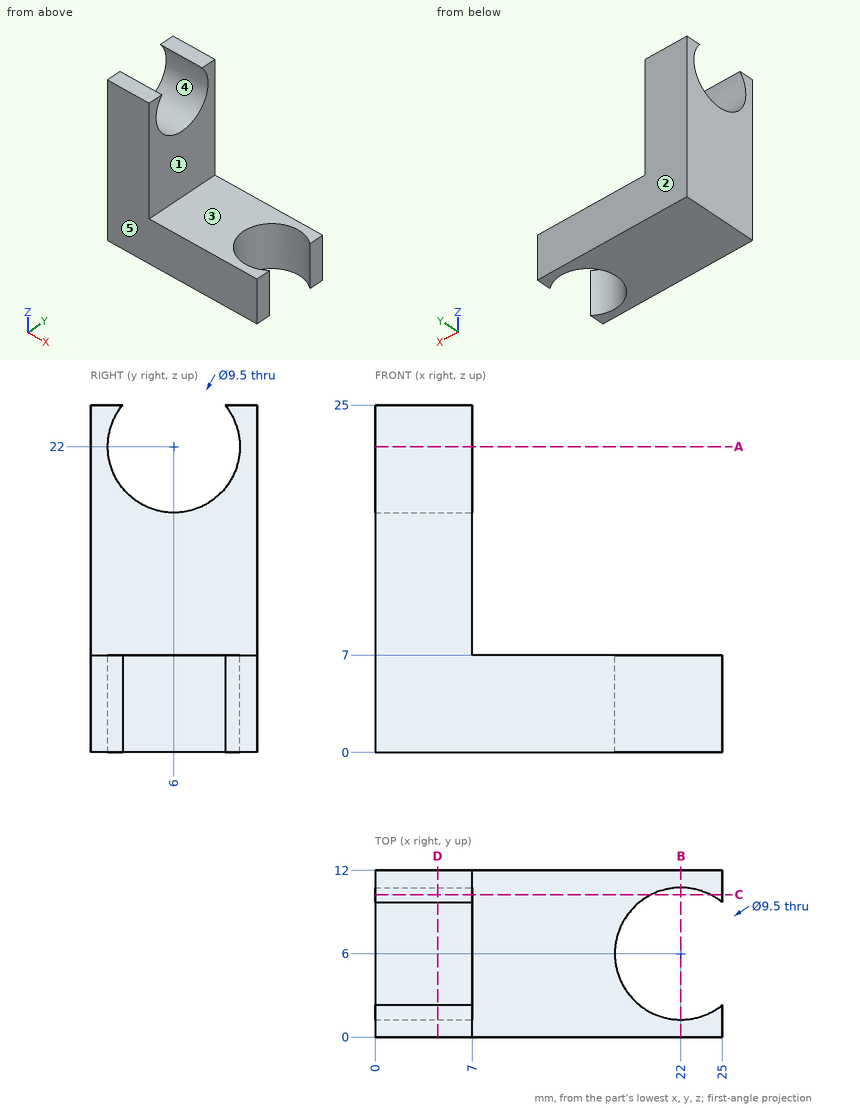
Answer from the drawing. Dimensions are ordinates in mm from the lowest x, y and z of the part. A direction names the side the tool comes from. Give positions to 0.01 mm unless a question says otherwise; leave off trailing zeros. Loops run counter-clockwise (first coordinate to the right, second up) from the corner with the lowest first, then second, coordinate; pieces in that order, holes last. Notation, with made-up numbers: (-22.75, 62) -> (15.25, 62) arc R17 ccw to (15.25, 84) -> close; hole circle Ø10 at (36, 55). An arc over 180 degrees is marked (long way). Use a Markdown table: item, result.
Q1. Section C-C, the plane y = 10.25 is taken. Determine the outline of the cut face in (x, z).
Solved:
| item | result |
|---|---|
| outline | (0, 0) -> (19.88, 0) -> (19.88, 7) -> (7, 7) -> (7, 19.88) -> (0, 19.88) -> close; (0, 24.12) -> (7, 24.12) -> (7, 25) -> (0, 25) -> close; (24.12, 0) -> (25, 0) -> (25, 7) -> (24.12, 7) -> close |
Q2. Section A-A, the plane z = 22 is taken. Determine the outline of the cut face in (x, y).
Solved:
| item | result |
|---|---|
| outline | (0, 0) -> (7, 0) -> (7, 1.25) -> (0, 1.25) -> close; (0, 10.75) -> (7, 10.75) -> (7, 12) -> (0, 12) -> close |
Q3. Find the intervals of material crossed by line 1 along Y through (x, z) = (3.25, 22); line 2 along X through (y, z) = (6, 17), in increasing order.
Solved:
| item | result |
|---|---|
| line 1 | y = 0 to 1.25, 10.75 to 12 |
| line 2 | x = 0 to 7 |
Q4. Section D-D, the plane x = 4.5 is taken. Determine the outline of the cut face in (y, z), then the cut area to 3 significant figures.
Solved:
| item | result |
|---|---|
| outline | (0, 0) -> (12, 0) -> (12, 25) -> (9.68, 25) arc R4.75 cw (long way) to (2.32, 25) -> (0, 25) -> close |
| area | 238 mm^2 |
Q5. Section B-B, the plane x = 22 is taken. Determine the outline of the cut face in (y, z), then the cut area to 3 significant figures.
Solved:
| item | result |
|---|---|
| outline | (0, 0) -> (1.25, 0) -> (1.25, 7) -> (0, 7) -> close; (10.75, 0) -> (12, 0) -> (12, 7) -> (10.75, 7) -> close |
| area | 17.5 mm^2 |
Q6. Each of these flat-tipped pins is pushed along its axis until it touches: pin 1 (4 mm diameter, centred on x = 21.5, y = 3, fed in from +Z); pin 2 (3 mm diameter, centred on y = 1.5, z = 16, fed in from +X). Where does it stop, or does it pass through?
Solved:
| item | result |
|---|---|
| pin 1 | stops at z = 7 |
| pin 2 | stops at x = 7 |
Q7. A tool of negligible diameter and unlimited length cuts with its end or side. For the marked faces 1 and 2, from which of +Z, -Z, +X, -X, +Y, -Y can it reach the whole face along a straight path? Write none if from no direction.
Solved:
| item | result |
|---|---|
| face 1 | +Z, +X, +Y, -Y |
| face 2 | +Z, -Z, +X, -X, +Y |
Q8. Determine the mould class of the marked faces 3, 4 and 5 for opening direction Y: pulls with the +Y half, pulls with the -Y half, needs draft (parallel to the pull), parting line crosses it, or undercut.
Solved:
| item | result |
|---|---|
| face 3 | needs draft |
| face 4 | undercut |
| face 5 | pulls with the -Y half |
